from build123d import *

# Parameters (mm, degrees)
F0_W     = 85.06
F0_H     = 63.2
F1_DEPTH = 5
F2_W     = 85.06
F2_H     = 63.2
F2_W_2   = 77.40441
F2_H_2   = 56.148566
F3_DEPTH = 16
F4_W     = 10.2
F4_H     = 12
F5_DEPTH = 25
F6_W     = 13
F6_H     = 12
F7_DEPTH = 3.827795
F8_R     = 3.75
F8_R_2   = 1
F8_R_3   = 1.25
F9_DEPTH = 5


with BuildPart() as f1:
    # F0 (on Top) → F1 (new body)
    with BuildSketch(Plane.XY):
        Rectangle(F0_W, F0_H)
    extrude(amount=F1_DEPTH)

    # F2 (on face) → F3 (join)
    with BuildSketch(Plane.XY.offset(5)):
        Rectangle(F2_W, F2_H)
        Rectangle(F2_W_2, F2_H_2, mode=Mode.SUBTRACT)
    extrude(amount=F3_DEPTH)

    # F4 (on face) → F5 (cut)
    with BuildSketch(Plane.YZ.offset(42.53)):
        with Locations((19.5, 11)):
            Rectangle(F4_W, F4_H)
    extrude(amount=-F5_DEPTH, mode=Mode.SUBTRACT)

    # F6 (on face) → F7 (cut, through all)
    with BuildSketch(Plane.YZ.offset(42.53)):
        with Locations((-15.1, 10.857148)):
            Rectangle(F6_W, F6_H)
    extrude(amount=-F7_DEPTH, mode=Mode.SUBTRACT)

    # F8 (on face) → F9 (join)
    with BuildSketch(Plane.XY.offset(5)):
        with Locations((-28.422205, 13.094283)):
            Circle(F8_R)
        with Locations((-28.422205, 13.094283)):
            Circle(F8_R_2, mode=Mode.SUBTRACT)
        with Locations((-29.664541, -4.354283)):
            Circle(F8_R)
        with Locations((-29.664541, -4.354283)):
            Circle(F8_R_3, mode=Mode.SUBTRACT)
        with Locations((7.469576, 16.546624)):
            Circle(F8_R)
        with Locations((7.469576, 16.546624)):
            Circle(F8_R_3, mode=Mode.SUBTRACT)
        with Locations((7.469576, -5.314252)):
            Circle(F8_R)
        with Locations((7.469576, -5.314252)):
            Circle(F8_R_3, mode=Mode.SUBTRACT)
    extrude(amount=F9_DEPTH)


solid = f1.part
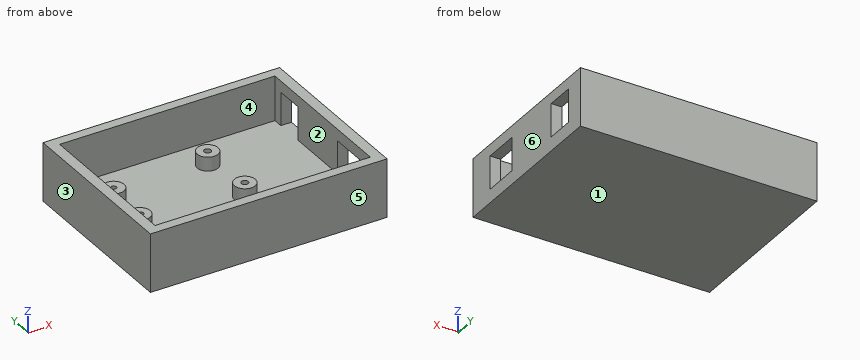
Could you check a few things on this model? Use its own coordinates, in mm. Face numbers are marked on the shaded views. A direction names the side the tool comes from. Give positions to 0.01 mm unless a question says otherwise; leave off trailing zeros. Order: outer loops, then holes, each group sorted by start corner. A loop starts at its lowest first (then second) coordinate and runs counter-clockwise, first axis right, second up.
Item 1: If we section it at C-C, the plane z = 14.25: Write out the boundary of the cut face in (x, y), plus the area to 3 significant figures.
Item 2: If we mould it in two halves opening along X, with no side actions, what happens to the marked faces 3, 4, 5 and 6? For each: pulls with the +X half, pulls with the -X half, needs draft (parallel to the pull), parting line crosses it, or undercut.
Item 3: I need wall thicknesses on line 1 (X direction, y = -24, z = 6.25); line 2 (Y direction, x = -28, z = 20); line 3 (Z direction, x = 15, y = -3). Which ranges of each line are inside material? Lowest first, please.
Item 4: If we section it at D-D, the plane x = -35: Write out the boundary of the cut face in (y, z), plus the area to 3 significant figures.
Item 5: For the marked faces 1 and 2, which set-ups out of +Z, -Z, +X, -X, +Y, -Y let a thin tool reach every point of the face, with its end or its side?
Item 6: If we section it at B-B, the plane z = 7.5: Count the separate pieces of the cut face and the enclosed holes in it, plus the area to 3 significant figures.
Item 7: I'm going to push flat-ended pins straight in: pin 1 (10 mm diameter, centred on x = 7.5, y = 16, fed in from +Z); pin 2 (4 mm diameter, centred on x = -9, y = -25, fed in from +Z). Where does each tip first touch, or does it pass through?
Item 8: If we section it at A-A, the plane y = -16: Write out the boundary of the cut face in (x, z), plus the area to 3 significant figures.
Values:
1. outline: (-42.53, -31.6) - (42.53, -31.6) - (42.53, -21.6) - (38.7, -21.6) - (38.7, -28.07) - (-38.7, -28.07) - (-38.7, 28.07) - (38.7, 28.07) - (38.7, 24.6) - (42.53, 24.6) - (42.53, 31.6) - (-42.53, 31.6) - close; (38.7, -8.6) - (42.53, -8.6) - (42.53, 14.4) - (38.7, 14.4) - close
1. area: 941 mm2
2. face 3: pulls with the -X half
2. face 4: undercut
2. face 5: needs draft
2. face 6: pulls with the +X half
3. line 1: x = -42.53 to -38.7, 38.7 to 42.53
3. line 2: y = -31.6 to -28.07, 28.07 to 31.6
3. line 3: z = 0 to 5
4. outline: (-31.6, 0) - (31.6, 0) - (31.6, 21) - (28.07, 21) - (28.07, 5) - (-28.07, 5) - (-28.07, 21) - (-31.6, 21) - close
4. area: 429 mm2
5. face 1: -Z, +X, -X, +Y, -Y
5. face 2: +Z
6. separate pieces: 6
6. enclosed holes: 4
6. area: 1,100 mm2
7. pin 1: stops at z = 10
7. pin 2: stops at z = 5
8. outline: (-42.53, 0) - (42.53, 0) - (42.53, 4.86) - (38.7, 4.86) - (38.7, 5) - (-38.7, 5) - (-38.7, 21) - (-42.53, 21) - close; (38.7, 16.86) - (42.53, 16.86) - (42.53, 21) - (38.7, 21) - close
8. area: 502 mm2
